The model under review builds one solid part; all positions refer to its coordinate system, in mm. A direction names the side the tool comes from. Coordinates: 2 decimals unless noted, no trailing zeros. Order: outer loops, then holes, each group sorted by start corner. A loop starts at its lowest first (then second) coordinate and runs counter-clockwise, first axis right, second up. Notation, with made-up numbers: M 40,25 L 78,25 A21 cw 78,64 Z; hole C 9,-40 d7. An arc over 180 degrees is marked long. One line per item, written item: value.
```python
from build123d import *

# Parameters (mm, degrees)
SKETCH_1_W             = 1
SKETCH_1_H             = 0.8
EXTRUDE_1_DEPTH        = 40
CUT_EXTRUDE_1_DEPTH    = 55
SKETCH_3_R             = 1.8
CUT_EXTRUDE_2_DEPTH    = 0.8
MOVE_FACE_2_BY         = 60
PATTERN_LINEAR_1_COUNT = 5
PATTERN_LINEAR_1_PITCH = 15


with BuildPart() as part:
    # 草图1 → 凸台-拉伸1 (new body)
    with BuildSketch(Plane.XY):
        with Locations((-3.159883721, 0.568023256)):
            Rectangle(SKETCH_1_W, SKETCH_1_H)
        Polygon((-0.159883721, -3.331976744), (-0.159883721, 1.468023256), (-2.659883721, 1.468023256), (-2.659883721, 0.968023256), (-2.659883721, 0.168023256), (-2.659883721, -3.331976744), align=None)
        Polygon((2.340116279, 0.968023256), (2.340116279, 1.468023256), (-0.159883721, 1.468023256), (-0.159883721, -3.331976744), (2.340116279, -3.331976744), (2.340116279, 0.168023256), align=None)
        with Locations((2.840116279, 0.568023256)):
            Rectangle(SKETCH_1_W, SKETCH_1_H)
    extrude(amount=EXTRUDE_1_DEPTH)

    # 草图2 → 切除-拉伸1 (cut)
    with BuildSketch(Plane(origin=(0, 1.468023256, 0), x_dir=(1, 0, 0), z_dir=(0, 1, 0))):
        with BuildLine():
            ThreePointArc((-0.159883721, -3.8), (-1.359883721, -5), (-0.159883721, -6.2))
            Line((-0.159883721, -6.2), (-0.159883721, -3.8))
        make_face()
        with BuildLine():
            Line((-0.159883721, -3.8), (-0.159883721, -6.2))
            ThreePointArc((-0.159883721, -6.2), (0.688644416, -5.848528137), (1.040116279, -5))
            ThreePointArc((1.040116279, -5), (0.688644416, -4.151471863), (-0.159883721, -3.8))
        make_face()
        with BuildLine():
            ThreePointArc((-1.359883721, -20), (-1.008411858, -20.848528137), (-0.159883721, -21.2))
            Line((-0.159883721, -21.2), (-0.159883721, -20))
            Line((-0.159883721, -20), (-1.359883721, -20))
        make_face()
        with BuildLine():
            Line((-0.159883721, -20), (-0.159883721, -21.2))
            ThreePointArc((-0.159883721, -21.2), (0.688644416, -20.848528137), (1.040116279, -20))
            Line((1.040116279, -20), (-0.159883721, -20))
        make_face()
        with BuildLine():
            Line((-1.359883721, -20), (-0.159883721, -20))
            Line((-0.159883721, -20), (-0.159883721, -18.8))
            ThreePointArc((-0.159883721, -18.8), (-1.008411858, -19.151471863), (-1.359883721, -20))
        make_face()
        with BuildLine():
            Line((-0.159883721, -18.8), (-0.159883721, -20))
            Line((-0.159883721, -20), (1.040116279, -20))
            ThreePointArc((1.040116279, -20), (0.688644416, -19.151471863), (-0.159883721, -18.8))
        make_face()
        with BuildLine():
            ThreePointArc((-0.159883721, -33.8), (-1.359883721, -35), (-0.159883721, -36.2))
            Line((-0.159883721, -36.2), (-0.159883721, -35))
            Line((-0.159883721, -35), (-0.159883721, -33.8))
        make_face()
        with BuildLine():
            Line((-0.159883721, -35), (-0.159883721, -36.2))
            ThreePointArc((-0.159883721, -36.2), (0.688644416, -35.848528137), (1.040116279, -35))
            ThreePointArc((1.040116279, -35), (0.688644416, -34.151471863), (-0.159883721, -33.8))
            Line((-0.159883721, -33.8), (-0.159883721, -35))
        make_face()
    cut_extrude_1 = extrude(amount=-CUT_EXTRUDE_1_DEPTH, mode=Mode.SUBTRACT)

    # 草图3 → 切除-拉伸2 (cut)
    with BuildSketch(Plane(origin=(0, 1.468023256, 0), x_dir=(1, 0, 0), z_dir=(0, 1, 0))):
        with Locations(Location((-0.159883721, -35, 0), (0, 0, 270))):
            Circle(SKETCH_3_R)
        with Locations(Location((-0.159883721, -20, 0), (0, 0, 270))):
            Circle(SKETCH_3_R)
        with Locations(Location((-0.159883721, -5, 0), (0, 0, 270))):
            Circle(SKETCH_3_R)
    cut_extrude_2 = extrude(amount=-CUT_EXTRUDE_2_DEPTH, mode=Mode.SUBTRACT)

    # Move Face 2: a face moved outward by 60.0
    extrude(part.faces().sort_by_distance((-0.159883721, -0.838226744, 40))[0], amount=MOVE_FACE_2_BY, dir=(0, 0, 1))

    # 阵列(线性)1: 切除-拉伸1, 切除-拉伸2 ×5
    with Locations(*[(0, 0, i * PATTERN_LINEAR_1_PITCH) for i in range(1, PATTERN_LINEAR_1_COUNT)]):
        add(cut_extrude_1, mode=Mode.SUBTRACT)
        add(cut_extrude_2, mode=Mode.SUBTRACT)


solid = part.part
```
(1) We need section A-A, the plane y = -2.2. State the section outline as (x, z) points, plus the area to 3 significant figures.
Geometry results:
outline: M -2.66,0 L 2.34,0 L 2.34,100 L -2.66,100 Z; hole C -0.16,5 d2.4; hole C -0.16,20 d2.4; hole C -0.16,35 d2.4; hole C -0.16,50 d2.4; hole C -0.16,65 d2.4; hole C -0.16,80 d2.4; hole C -0.16,95 d2.4
area: 468 mm2
(2) For L1, parallel to X at y = 1.2, z = 50; L2, parallel to X at y = -1.75, z = 43.5; L3, parallel to Y at x = 2.5, z = 65, list the stretches that pass through material, from the lowest coordinate up.
Geometry results:
L1: x = -2.66 to -1.96, 1.64 to 2.34
L2: x = -2.66 to 2.34
L3: y = 0.17 to 0.97
(3) We need section B-B, the plane z = 25. State the section outline as (x, y) points.
Geometry results:
outline: M -3.66,0.17 L -2.66,0.17 L -2.66,-3.33 L 2.34,-3.33 L 2.34,0.17 L 3.34,0.17 L 3.34,0.97 L 2.34,0.97 L 2.34,1.47 L -2.66,1.47 L -2.66,0.97 L -3.66,0.97 Z
(4) Insertion check: pin 1 Ø3 at (x, z) = (-0.16, 80) entering from +Y; pin 2 Ø1.1 at (x, z) = (3, 66) entering from +Y; pin 3 Ø1 at (y, z) = (-0.5, 37.5) entering from -X; pin 4 Ø2 at (x, z) = (-0.16, 20) entering from +Y. Each pin has a flat end and moves straight along its axis. Give the tip position at first contact, or say it passes through.
Geometry results:
pin 1: stops at y = 0.67
pin 2: stops at y = 0.97
pin 3: stops at x = -2.66
pin 4: passes through
(5) Tool access review of faces 4 (the flat face through (2.34, -2, 49)), 5 (the flat face through (1, -3.332, 49)), 6 (the cylindrical face through (-1.757, 1.074, 50.831)), 7 (the flat face through (-2.66, -2, 49)): name each direction out of +Z, -Z, +X, -X, +Y, -Y from which nothing blocks a thin tool from reaching the whole face with its end or side.
Geometry results:
face 4: +Z, -Z, +X, -Y
face 5: +Z, -Z, +X, -X, -Y
face 6: +Y
face 7: +Z, -Z, -X, -Y
(6) Mouldability with a two-part tool opening along Z and no side actions: class faces 1 (the flat face through (2, 1.468, 49)), 2 (the flat face through (0, -1, 100)), 3 (the cylindrical face through (-0.1, 1.1, 93.2)) as +Z half, -Z half, draft (parallel to the pull), parting line (faces both ways), or undercut.
Geometry results:
face 1: draft
face 2: +Z half
face 3: undercut
